Part model, mm, in its own coordinate system. A direction names the side the tool comes from. Coordinates: 2 decimals unless noted, no trailing zeros. Loops run counter-clockwise (first coordinate to the right, second up) from the corner with the lowest first, then second, coordinate; pieces in that order, holes last. Notation, with made-up numbers: (-8, -38) - (0, -38) arc R13 cw to (0, -14) - close; hole circle Ø11 at (63.25, -40). An arc over 180 degrees is marked (long way). Use a Markdown table: item, result. Add a question column.
1. Band-saw the part on D-D, the plane z = -39. Give the cut face in (x, y), plus the area to 3 significant figures.
2. Drop flat-ended pins along their axis: pin 1 (23 mm diameter, centred on x = -61, y = -15.5, fed in from +Z); pin 2 (12 mm diameter, centred on x = -1.5, z = -20.5, fed in from -Y); pin 3 (1.5 mm diameter, centred on y = -35, z = -64, fed in from +X). Give the stop position or say it passes through.
3. Band-saw the part on A-A, the plane y = -42. Give the cut face in (x, z).
4. Band-saw the part on B-B, the plane z = 0. Give the cut face in (x, y).
5. Pull direction Z, two halves, no side cores. Call faces 1 (the flat face through (63, -19, 10.16)), 2 (the cylindrical face through (-76.574, -37.567, -58.715)), 3 (the flat face through (-79, -76.2, 22)): pulls with the +Z half, pulls with the -Z half, needs draft (parallel to the pull), parting line crosses it, or undercut.
6. Band-saw the part on C-C, the plane x = 0. Give the cut face in (y, z), plus the area to 3 significant figures.
7. Wall check: probe 1 along X at (y, z) = (-15.5, -37.5); probe 2 along Z at (x, y) = (0, -54.5); probe 3 along Z at (x, y) = (-69.5, -35.5). Give the ranges that are in metal, low to high. Write a range as [from, to].
8. 3-axis set-ups, long thin cutter, end or side, ignore diameter. For faces 4 (the flat face through (-10.16, -19, 63)), 5 (the flat face through (-1, 0, 1)), 6 (the flat face through (-1, -25.4, 1)): which of +Z, -Z, +X, -X, +Y, -Y reach the whole face in a straight line?
from build123d import *

# Parameters (mm, degrees)
F0_R     = 96.493777
F0_R_2   = 81.643771
F1_DEPTH = 76.2
F2_W     = 80.01
F2_H     = 20.32
F2_W_2   = 20.32
F2_H_2   = 80.01
F3_DEPTH = 25.4
F4_R     = 36.256565
F5_DEPTH = 25.4
F6_SIZE  = 25.4


with BuildPart() as f1:
    # F0 (on Front) → F1 (new body)
    with BuildSketch(Plane.XZ):
        Circle(F0_R)
        Circle(F0_R_2, mode=Mode.SUBTRACT)
    extrude(amount=F1_DEPTH)

    # F2 (on Front) → F3 (join)
    with BuildSketch(Plane.XZ):
        with Locations((-50.165, 0)):
            Rectangle(F2_W, F2_H)
        with Locations((0, -50.165)):
            Rectangle(F2_W_2, F2_H_2)
        with Locations((50.165, 0)):
            Rectangle(F2_W, F2_H)
        with Locations((0, 50.165)):
            Rectangle(F2_W_2, F2_H_2)
    extrude(amount=F3_DEPTH)

    # F4 (on Front) → F5 (join)
    with BuildSketch(Plane.XZ):
        Circle(F4_R)
    extrude(amount=F5_DEPTH)

    # F6
    f6_edges = [f1.edges().sort_by_distance(p)[0] for p in [
        (81.484957, -25.4, 5.089901),
        (0, -25.4, 81.643771),
        (-81.643771, -25.4, 0),
        (0, -25.4, -81.643771),
        (81.484957, -25.4, -5.089901),
    ]]
    chamfer(f6_edges, length=F6_SIZE)


solid = f1.part
Geometry check:
| question | item | result |
|---|---|---|
| 1 | outline | (-88.26, -76.2) - (-71.73, -76.2) - (-71.73, 0) - (-88.26, 0) - close; (-10.16, -25.4) - (10.16, -25.4) - (10.16, 0) - (-10.16, 0) - close; (71.73, -76.2) - (88.26, -76.2) - (88.26, 0) - (71.73, 0) - close |
| 1 | area | 3,040 mm^2 |
| 2 | pin 1 | stops at z = 82.83 |
| 2 | pin 2 | stops at y = -25.4 |
| 2 | pin 3 | stops at x = 72.87 |
| 3 | outline | circle Ø192.99 at (0, 0); hole (-81.01, -10.16) arc R81.64 ccw to (-10.16, -81.01) - (-10.16, -72.13) arc R72.84 ccw to (10.16, -72.13) - (10.16, -81.01) arc R81.64 ccw to (81.01, -10.16) - (72.13, -10.16) arc R72.84 ccw to (72.13, 10.16) - (81.01, 10.16) arc R81.64 ccw to (10.16, 81.01) - (10.16, 72.13) arc R72.84 ccw to (-10.16, 72.13) - (-10.16, 81.01) arc R81.64 ccw to (-81.01, 10.16) - (-72.13, 10.16) arc R72.84 ccw to (-72.13, -10.16) - close |
| 4 | outline | (-96.49, -76.2) - (-81.64, -76.2) - (-81.64, -50.8) - (-56.24, -25.4) - (56.24, -25.4) - (81.64, -50.8) - (81.64, -76.2) - (96.49, -76.2) - (96.49, 0) - (-96.49, 0) - close |
| 5 | face 1 | undercut |
| 5 | face 2 | parting line crosses it |
| 5 | face 3 | needs draft |
| 6 | outline | (-76.2, -96.49) - (0, -96.49) - (0, 96.49) - (-76.2, 96.49) - (-76.2, 81.64) - (-50.8, 81.64) - (-25.4, 56.24) - (-25.4, -56.24) - (-50.8, -81.64) - (-76.2, -81.64) - close |
| 6 | area | 7,060 mm^2 |
| 7 | probe 1 | x = [-88.91, -72.52], [-10.16, 10.16], [72.52, 88.91] |
| 7 | probe 2 | z = [-96.49, -81.64], [81.64, 96.49] |
| 7 | probe 3 | z = [-66.94, -42.84], [-10.16, 10.16], [42.84, 66.94] |
| 8 | face 4 | +Y, -Y |
| 8 | face 5 | +Z, -Z, +X, -X, +Y |
| 8 | face 6 | -Y |
